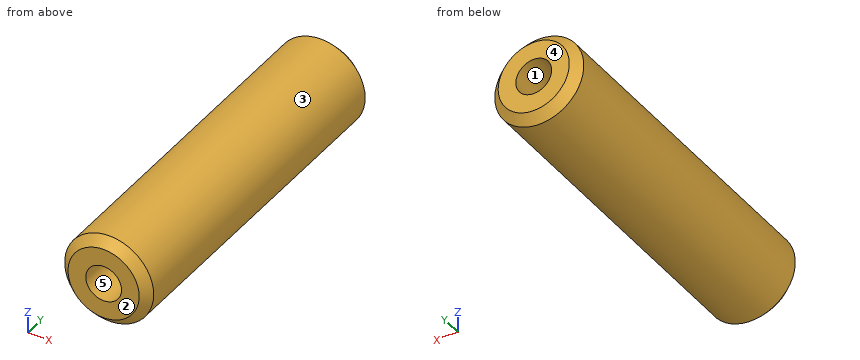
```python
from build123d import *

# Parameters (mm, degrees)
SKETCH1_R                   = 6.35
BOSS_EXTRUDE1_DEPTH         = 50.8
CHAMFER1_SIZE               = 1.27
F_1_4_20_TAPPED_HOLE1_D     = 5.1054
F_1_4_20_TAPPED_HOLE1_DEPTH = 16.51
F_1_4_20_TAPPED_HOLE1_TIP   = 1.533816902
F_1_4_20_TAPPED_HOLE2_D     = 5.1054
F_1_4_20_TAPPED_HOLE2_DEPTH = 16.51
F_1_4_20_TAPPED_HOLE2_TIP   = 1.533816902


with BuildPart() as part:
    # Sketch1 → Boss-Extrude1 (new body)
    with BuildSketch(Plane(origin=(0, 0, 0), x_dir=(1, 0, 0), z_dir=(0, 1, 0))):
        Circle(SKETCH1_R)
    extrude(amount=BOSS_EXTRUDE1_DEPTH)

    # Chamfer1
    chamfer1_edges = [part.edges().sort_by_distance(p)[0] for p in [
        (-6.35, 0, 0),
        (-6.35, 50.8, 0),
    ]]
    chamfer(chamfer1_edges, length=CHAMFER1_SIZE)

    # 1/4-20 Tapped Hole1
    with Locations(Plane(origin=(0, 0, 0), x_dir=(-1, 0, 0), z_dir=(0, -1, 0))):
        with Locations((0, 0)):
            Hole(F_1_4_20_TAPPED_HOLE1_D / 2, depth=F_1_4_20_TAPPED_HOLE1_DEPTH)
            with Locations((0, 0, -(F_1_4_20_TAPPED_HOLE1_DEPTH + F_1_4_20_TAPPED_HOLE1_TIP / 2))):  # 118° drill point
                Cone(0, F_1_4_20_TAPPED_HOLE1_D / 2, F_1_4_20_TAPPED_HOLE1_TIP, mode=Mode.SUBTRACT)

    # 1/4-20 Tapped Hole2
    with Locations(Plane(origin=(0, 50.8, 0), x_dir=(1, 0, 0), z_dir=(0, 1, 0))):
        with Locations((0, 0)):
            Hole(F_1_4_20_TAPPED_HOLE2_D / 2, depth=F_1_4_20_TAPPED_HOLE2_DEPTH)
            with Locations((0, 0, -(F_1_4_20_TAPPED_HOLE2_DEPTH + F_1_4_20_TAPPED_HOLE2_TIP / 2))):  # 118° drill point
                Cone(0, F_1_4_20_TAPPED_HOLE2_D / 2, F_1_4_20_TAPPED_HOLE2_TIP, mode=Mode.SUBTRACT)


solid = part.part
```
The listing builds one solid part. Answer for the finished solid, in the listing's coordinates (mm). Face numbers are marked on the shaded views. A direction names the side the tool comes from. Coordinates: 2 decimals unless noted, no trailing zeros. Write each loop counter-clockwise with the first axis right and the second up, starting at its lowest first coordinate (ties: lowest second). Pieces come first, ordered by that corner, then holes. Notation, with made-up numbers: (-34.5, 66.5) - (-22.5, 66.5) arc R31 ccw to (-22.5, 101.5) - close; hole circle Ø9 at (32, -30.75). An arc over 180 degrees is marked (long way). Return JSON: item names as keys, results as strings. Group by question number.
1. Determine the mould class of the marked faces 1, 2 and 3 for opening direction Z: released by +Z, released by -Z, zero draft, split by the parting line, or undercut.
2. Which of the six approach directions +Z, -Z, +X, -X, +Y, -Y give full straight-line access (tool end or side, diameter ignored) to the marked faces 4 and 5?
3. A cutting plane is placed at A-A, the plane y = 41.5. Determine the outline of the cut face in (x, z), plus the area to 3 significant figures.
4. A cutting plane is placed at B-B, the plane y = 31. Determine the outline of the cut face in (x, z).
5. Given pin 1 (1.5 mm diameter, centred on y = 40.5, z = -2.5, fed in from +X); pin 2 (4 mm diameter, centred on x = -3, y = 28.5, fed in from +Z); pin 3 (4.5 mm diameter, centred on x = 0, z = 0, fed in from -Y), each flat-ended and moving along its own axis, determine where each tip first touches the part or whether it passes through.
6. Straight lines are drawn through the part: L1, parallel to Z at x = 0, y = 6.5; L2, parallel to X at y = 6.5, z = -1.25; L3, parallel to Z at x = 2.25, y = 48.5. For each, find the intervals that lie inside material, in ascending order.
Ans:
{
 "1": {"face 1": "undercut", "face 2": "zero draft", "face 3": "split by the parting line"},
 "2": {"face 4": "+Z, -Z, +X, -X, +Y", "face 5": "-Y"},
 "3": {"outline": "circle Ø12.7 at (0, 0); hole circle Ø5.11 at (0, 0)", "area": "106 mm²"},
 "4": {"outline": "circle Ø12.7 at (0, 0)"},
 "5": {"pin 1": "x = 6.1", "pin 2": "z = 6.27", "pin 3": "y = 16.69"},
 "6": {"L1": "-6.35 to -2.55, 2.55 to 6.35", "L2": "-6.23 to -2.23, 2.23 to 6.23", "L3": "-5.94 to -1.21, 1.21 to 5.94"}
}
